Work out the finished part from the listing and answer in its coordinate system (mm). Round coordinates to 2 decimals unless told otherwise and drop trailing zeros. Write each loop counter-clockwise with the first axis right and the second up, starting at its lowest first coordinate (ties: lowest second). Pieces come first, ordered by that corner, then holes. Notation, with made-up numbers: (-33.5, 34) -> (-23.5, 34) arc R24 ccw to (-23.5, 72) -> close; hole circle Ø1 at (46.25, -38). An arc over 180 degrees is marked (long way). One line per item, written item: value.
```python
from build123d import *

# Parameters (mm, degrees)
F0_W     = 118.4896603227
F0_H     = 130.4209120572
F1_DEPTH = 25
F2_D     = 10


with BuildPart() as f1:
    # F0 (on Top) → F1 (new body)
    with BuildSketch(Plane.XY):
        with Locations((3.7028007209, -2.8799604625)):
            Rectangle(F0_W, F0_H)
    extrude(amount=F1_DEPTH)

    # F2 (through all)
    with Locations(Plane(origin=(0, 0, 0), x_dir=(1, 0, 0), z_dir=(0, 0, -1))):
        with Locations((-45.2564693987, -49.9878264964), (4.52564843, -51.2220934033), (53.484916687, -49.1649806499), (52.2506535053, 0), (51.0163828731, 58.2162737846), (4.1142245755, 58.6276985705), (-44.8450483382, 58.2162737846), (-45.2564693987, 0)):
            Hole(F2_D / 2)


solid = f1.part
```
(1) Find section B-B on z = 15.5. Give the number of separate pieces and of enclosed holes in the cut face, plus the area to 3 significant figures.
Reported:
separate pieces: 1
enclosed holes: 8
area: 14,800 mm2
(2) Find section A-A on y = 0. Give the vertices of the cut face in (x, z), plus the area to 3 significant figures.
Reported:
outline: (-55.54, 0) -> (-50.26, 0) -> (-50.26, 25) -> (-55.54, 25) -> close; (-40.26, 0) -> (47.25, 0) -> (47.25, 25) -> (-40.26, 25) -> close; (57.25, 0) -> (62.95, 0) -> (62.95, 25) -> (57.25, 25) -> close
area: 2,460 mm2
(3) For a pull along X with two mould halves and no side action, classify faces 1 (the face through (3, -2, 25)), 2 (the face through (62.948, -4, 12)), 3 (the face through (5.177, 46.265, 12.675)) as pulls with the +X half, pulls with the -X half, needs draft (parallel to the pull), parting line crosses it, or undercut.
Reported:
face 1: needs draft
face 2: pulls with the +X half
face 3: undercut
(4) A flat-ended cylindrical pin translates along its axis: pin 1 Ø6 at (x, y) = (53.48, 49.16) entering from -Z. Find the tip coordinate at first contact, or state that the pin passes through.
Reported:
pin 1: passes through
(5) Consider probe 1 along Y at (x, z) = (-45, 11); probe 2 along Y at (x, z) = (-46, 6.75); probe 3 along X at (y, z) = (-59.5, 12.5). Determine where each line is inside the solid, lowest interval first.
Reported:
probe 1: y = -68.09 to -63.21, -53.22 to -4.99, 4.99 to 44.99, 54.98 to 62.33
probe 2: y = -68.09 to -63.08, -53.35 to -4.94, 4.94 to 45.04, 54.93 to 62.33
probe 3: x = -55.54 to -49.68, -40.01 to -0.81, 9.04 to 46.18, 55.85 to 62.95
